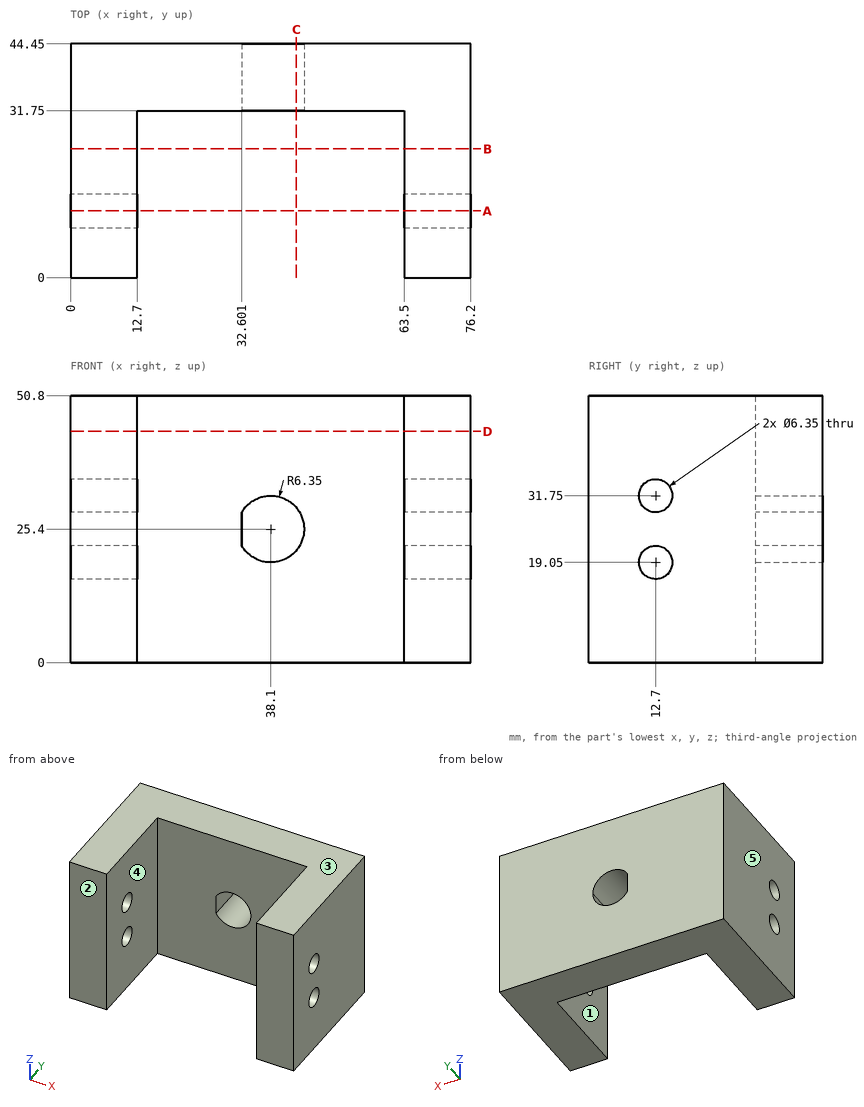
Geometry: see drawing. Coordinates: mm, zero at the bounding-box minimum. A direction names the side the tool comes from. Round coordinates to 2 decimals unless told otherwise and drop trailing zeros. Write each loop counter-clockwise with the first axis right and the second up, starting at its lowest first coordinate (ties: lowest second). Pieces come first, ordered by that corner, then holes. Notation, with made-up numbers: (-3, -1.5) -> (40, -1.5) arc R18 cw to (40, 13.5) -> close; hole circle Ø10 at (11.25, -13). An arc over 180 degrees is marked (long way). Answer as CSV lines item,"result".
1. Mould query, pull axis X, two halves, no side actions, for the marked faces 3, 4 and 5. Classes: +X half, -X half, draft (parallel to the pull), parting line (faces both ways), or undercut.
Geometry says:
face 3,"draft"
face 4,"undercut"
face 5,"-X half"
2. Section C-C (x = 43). Return the cut outline in (y, z).
Geometry says:
outline,"(31.75, 0) -> (44.45, 0) -> (44.45, 21.36) -> (31.75, 21.36) -> close; (31.75, 29.44) -> (44.45, 29.44) -> (44.45, 50.8) -> (31.75, 50.8) -> close"
3. Contact query for flat-ended pins moving along their axis: P1, Ø5.5, axis at y = 12.7, z = 19.05, coming from the +X side; P2, Ø2, axis at x = 51, z = 9, coming from the -Y side. Output: stop coordinate, or through.
Geometry says:
P1,"passes through"
P2,"stops at y = 31.75"
4. Section B-B (y = 24.5). Return the cut outline in (x, z).
Geometry says:
outline,"(0, 0) -> (12.7, 0) -> (12.7, 50.8) -> (0, 50.8) -> close; (63.5, 0) -> (76.2, 0) -> (76.2, 50.8) -> (63.5, 50.8) -> close"
5. Reachability of the marked faces 1 and 2 from +Z, -Z, +X, -X, +Y, -Y: full face, straight path, thin tool, end or side. Return the list, or none.
Geometry says:
face 1,"+Z, -Z, -Y"
face 2,"+Z, -Z, +X, -X, -Y"
6. Ray query, L1, parallel to Z at x = 9, y = 13; L2, parallel to X at y = 12, z = 26.5; L3, parallel to X at y = 35.5, z = 28.5. Return the intervals inside material, ascending. Write a range as [from, to].
Geometry says:
L1,"z = [0, 15.89], [22.21, 28.59], [34.91, 50.8]"
L2,"x = [0, 12.7], [63.5, 76.2]"
L3,"x = [0, 32.6], [43.64, 76.2]"
7. Section A-A (y = 12.7). Return the cut outline in (x, z) (1 decimal), plus the area to 3 significant figures.
Geometry says:
outline,"(0, 0) -> (12.7, 0) -> (12.7, 15.9) -> (0, 15.9) -> close; (0, 22.2) -> (12.7, 22.2) -> (12.7, 28.6) -> (0, 28.6) -> close; (0, 34.9) -> (12.7, 34.9) -> (12.7, 50.8) -> (0, 50.8) -> close; (63.5, 0) -> (76.2, 0) -> (76.2, 15.9) -> (63.5, 15.9) -> close; (63.5, 22.2) -> (76.2, 22.2) -> (76.2, 28.6) -> (63.5, 28.6) -> close; (63.5, 34.9) -> (76.2, 34.9) -> (76.2, 50.8) -> (63.5, 50.8) -> close"
area,"968 mm^2"
8. Section D-D (z = 44). Return the cut outline in (x, y).
Geometry says:
outline,"(0, 0) -> (12.7, 0) -> (12.7, 31.75) -> (63.5, 31.75) -> (63.5, 0) -> (76.2, 0) -> (76.2, 44.45) -> (0, 44.45) -> close"
